```python
from build123d import *

# Parameters (mm, degrees)
SKETCH_1_R          = 80
SKETCH_1_R_2        = 5
EXTRUDE_1_DEPTH     = 2.5
SKETCH_2_R          = 1.5
CUT_EXTRUDE_1_DEPTH = 114.164702978


with BuildPart() as part:
    # 草图1 → 凸台-拉伸1 (new body)
    with BuildSketch(Plane.XY):
        Circle(SKETCH_1_R)
        Circle(SKETCH_1_R_2, mode=Mode.SUBTRACT)
        with BuildLine():
            Line((-3, 19.773719933), (-3, 69.93568474))
            ThreePointArc((-3, 69.93568474), (-60.621778265, 35), (-62.066079616, -32.369766158))
            Line((-62.066079616, -32.369766158), (-18.62454379, -7.288783755))
            ThreePointArc((-18.62454379, -7.288783755), (-17.320508076, 10), (-3, 19.773719933))
        make_face(mode=Mode.SUBTRACT)
        with BuildLine():
            Line((3, 19.773719933), (3, 69.93568474))
            ThreePointArc((3, 69.93568474), (60.621778265, 35), (62.066079616, -32.369766158))
            Line((62.066079616, -32.369766158), (18.62454379, -7.288783755))
            ThreePointArc((18.62454379, -7.288783755), (17.320508076, 10), (3, 19.773719933))
        make_face(mode=Mode.SUBTRACT)
        with BuildLine():
            Line((15.62454379, -12.484936178), (59.066079616, -37.565918581))
            ThreePointArc((59.066079616, -37.565918581), (0, -70), (-59.066079616, -37.565918581))
            Line((-59.066079616, -37.565918581), (-15.62454379, -12.484936178))
            ThreePointArc((-15.62454379, -12.484936178), (0, -20), (15.62454379, -12.484936178))
        make_face(mode=Mode.SUBTRACT)
    extrude(amount=EXTRUDE_1_DEPTH)

    # 草图2 → 切除-拉伸1 (cut, through all)
    with BuildSketch(Plane(origin=(0, 0, 0), x_dir=(-1, 0, 0), z_dir=(0, 0, -1))):
        with Locations((-7.000881354, -3.871389966)):
            Circle(SKETCH_2_R)
        with Locations((-3.871389966, 7.000881354)):
            Circle(SKETCH_2_R)
        with Locations((7.000881354, 3.871389966)):
            Circle(SKETCH_2_R)
        with Locations((3.871389966, -7.000881354)):
            Circle(SKETCH_2_R)
    extrude(amount=-CUT_EXTRUDE_1_DEPTH, mode=Mode.SUBTRACT)


solid = part.part
```
Source: CAD feature listing. Evaluate the final solid. Frame: model axes, mm. A direction names the side the tool comes from. Give positions to 0.01 mm unless a question says otherwise; leave off trailing zeros. Loops run counter-clockwise (first coordinate to the right, second up) from the corner with the lowest first, then second, coordinate; pieces in that order, holes last. Notation, with made-up numbers: (73.5, 62) -> (105.5, 62) arc R21 ccw to (105.5, 85) -> close; hole circle Ø6 at (-28, 3). An arc over 180 degrees is marked (long way). Use a Markdown table: item, result. Add a question column.
(1) Section query C-C (z = 1.15). Count the separate pieces of the cut face and the enclosed holes in it, then the cut area to 3 significant figures.
(2) First-contact query: pin 1 Ø1.5 at (y, z) = (-26, 2) entering from -X; pin 2 Ø1 at (x, z) = (-12.5, 2) entering from -Y; pin 3 Ø1.2 at (y, z) = (38, 1.5) entering from +X. Flat tips, straight axial feed; report the tip coordinate or a pass-through.
(3) Section query B-B (y = 0). Output: boundary loops of the cut face in (x, z).
(4) Section query A-A (x = 0). Output: boundary loops of the cut face in (y, z).
(5) Section query D-D (y = -68). Output: boundary loops of the cut face in (x, z).
(6) Ray query, line 1 (Y direction, x = -21, z = 0.9); line 2 (Y direction, x = -8, z = 0.2); line 3 (X direction, y = 30.5, z = 1.9). Return the intervals inside material, ascending.
(7) Pull-direction query (Y, two-part tool) for faces 3 (the face through (0.984, -69.993, 1.232)), 4 (the face through (-17.34, -78.1, 1.23)), 5 (the face through (0, -6, 0)); classes: +Y half, -Y half, draft (parallel to the pull), parting line (faces both ways), or undercut.
(8) Access query for faces 1 (the face through (37.04, -24.85, 1.23)), 2 (the face through (0, -6, 2.5)). Directions: +Z, -Z, +X, -X, +Y, -Y. A direction counts if a zero-diameter tool reaches every point of the face in a straight line with its end or side. Return the directions, or none.
Checked values:
| question | item | result |
|---|---|---|
| 1 | separate pieces | 1 |
| 1 | enclosed holes | 8 |
| 1 | area | 6,760 mm^2 |
| 2 | pin 1 | x = -75.91 |
| 2 | pin 2 | y = -79.09 |
| 2 | pin 3 | x = 70.72 |
| 3 | outline | (-80, 0) -> (-70, 0) -> (-70, 2.5) -> (-80, 2.5) -> close; (-20, 0) -> (-5, 0) -> (-5, 2.5) -> (-20, 2.5) -> close; (5, 0) -> (20, 0) -> (20, 2.5) -> (5, 2.5) -> close; (70, 0) -> (80, 0) -> (80, 2.5) -> (70, 2.5) -> close |
| 4 | outline | (-80, 0) -> (-70, 0) -> (-70, 2.5) -> (-80, 2.5) -> close; (-20, 0) -> (-5, 0) -> (-5, 2.5) -> (-20, 2.5) -> close; (5, 0) -> (80, 0) -> (80, 2.5) -> (5, 2.5) -> close |
| 5 | outline | (-42.14, 0) -> (-16.61, 0) -> (-16.61, 2.5) -> (-42.14, 2.5) -> close; (16.61, 0) -> (42.14, 0) -> (42.14, 2.5) -> (16.61, 2.5) -> close |
| 6 | line 1 | -77.19 to -66.78, -15.59 to -8.66, 66.78 to 77.19 |
| 6 | line 2 | -79.6 to -69.54, -18.33 to 2.75, 4.99 to 18.33, 69.54 to 79.6 |
| 6 | line 3 | -73.96 to -63.01, -3 to 3, 63.01 to 73.96 |
| 7 | face 3 | undercut |
| 7 | face 4 | parting line |
| 7 | face 5 | draft |
| 8 | face 1 | +Z, -Z |
| 8 | face 2 | +Z, +X, -X, +Y, -Y |
